Design review of the part built by this model. Coordinates are the model's own, in mm. A direction names the side the tool comes from. Give positions to 0.01 mm unless a question says otherwise; leave off trailing zeros. Write each loop counter-clockwise with the first axis right and the second up, starting at its lowest first coordinate (ties: lowest second). Pieces come first, ordered by that corner, then holes. Notation, with made-up numbers: (62, 20.5) -> (72, 20.5) arc R19 cw to (72, 39.5) -> close; hole circle Ø9 at (43.25, -17). An arc over 180 degrees is marked (long way). Put each result on its own line as item: value. Start each with the question number.
from build123d import *

# Parameters (mm, degrees)
F1_DEPTH        = 12.7
F3_DEPTH        = 25.4
F4_W            = 242.7691146731
F4_H            = 30.0364848226
F5_DEPTH        = 12.7
F6_R            = 14.6387815084
F7_DEPTH        = 25.4
F8_R            = 8.3487757397
F9_DEPTH        = 25.4
F11_DEPTH       = 5.08
F13_DEPTH       = 5.08
F15_D           = 8.8
F15_CSINK_D     = 17.92
F15_CSINK_ANGLE = 90


with BuildPart() as f1:
    # F0 (on Top) → F1 (new body)
    with BuildSketch(Plane.XY):
        with BuildLine():
            Line((-109.5926865071, 0), (109.5926865071, 0))
            ThreePointArc((109.5926865071, 0), (0, 109.5926865071), (-109.5926865071, 0))
        make_face()
    extrude(amount=F1_DEPTH)

    # F2 (on Top) → F3 (join)
    with BuildSketch(Plane.XY):
        with BuildLine():
            Line((-99.2360358279, 0), (99.2360358279, 0))
            ThreePointArc((99.2360358279, 0), (0, 99.2360358279), (-99.2360358279, 0))
        make_face()
    extrude(amount=F3_DEPTH)

    # F4 (on Top) → F5 (cut)
    with BuildSketch(Plane.XY):
        with Locations((-4.4899918139, -4.9826959148)):
            Rectangle(F4_W, F4_H)
    extrude(amount=F5_DEPTH, mode=Mode.SUBTRACT)

    # F6 (on Top) → F7 (join)
    with BuildSketch(Plane.XY):
        Circle(F6_R)
    extrude(amount=F7_DEPTH)

    # F8 (on Top) → F9 (cut)
    with BuildSketch(Plane.XY):
        Circle(F8_R)
    extrude(amount=F9_DEPTH, mode=Mode.SUBTRACT)

    # F10 (on Top) → F11 (cut)
    with BuildSketch(Plane.XY):
        with BuildLine():
            ThreePointArc((81.0422290099, 30.3221999213), (83.5344690722, 31.6522479843), (83.8168430896, 34.4630402733))
            ThreePointArc((83.8168430896, 34.4630402733), (71.7577369395, 55.3515268057), (54.6157974615, 72.3192851046))
            ThreePointArc((54.6157974615, 72.3192851046), (52.4026696923, 72.89779249), (50.4251048932, 71.7480782719))
            Line((50.4251048932, 71.7480782719), (22.4235640904, 35.1450000601))
            ThreePointArc((22.4235640904, 35.1450000601), (22.1166466893, 31.9933659242), (24.806293545, 30.3221999213))
            Line((24.806293545, 30.3221999213), (81.0422290099, 30.3221999213))
        make_face()
        with BuildLine():
            ThreePointArc((-4.9650533663, 33.315884659), (-2.6194064658, 32.1600273833), (-0.2580637548, 33.2834712068))
            Line((-0.2580637548, 33.2834712068), (36.3094015687, 78.8968902074))
            ThreePointArc((36.3094015687, 78.8968902074), (36.8765863049, 81.5111398441), (35.1316920138, 83.538784685))
            ThreePointArc((35.1316920138, 83.538784685), (-1.7558791181, 90.6083948589), (-38.3418575582, 82.1149577688))
            ThreePointArc((-38.3418575582, 82.1149577688), (-39.9894725562, 80.0980697861), (-39.4389206806, 77.5526101127))
            Line((-39.4389206806, 77.5526101127), (-4.9650533663, 33.315884659))
        make_face()
        with BuildLine():
            ThreePointArc((-28.6519128364, 30.3221999213), (-25.9512730857, 32.0158519826), (-26.2999293888, 35.1845032967))
            Line((-26.2999293888, 35.1845032967), (-53.425476113, 69.442529))
            ThreePointArc((-53.425476113, 69.442529), (-55.4614488813, 70.5635354057), (-57.6870926805, 69.8939458642))
            ThreePointArc((-57.6870926805, 69.8939458642), (-70.419089982, 57.0448603864), (-80.3456057092, 41.9231197982))
            ThreePointArc((-80.3456057092, 41.9231197982), (-80.3231983412, 39.1054090847), (-77.9741099322, 37.5492023498))
            ThreePointArc((-77.9741099322, 37.5492023498), (-71.346139634, 35.2966967191), (-66.4208829403, 30.3221999213))
            Line((-66.4208829403, 30.3221999213), (-28.6519128364, 30.3221999213))
        make_face()
    extrude(amount=F11_DEPTH, mode=Mode.SUBTRACT)

    # F12 (on Top) → F13 (cut)
    with BuildSketch(Plane.XY):
        with BuildLine():
            ThreePointArc((-89.5017917801, 37.8877817543), (-64.6761122502, 72.5469175245), (-27.4057276817, 93.2468810649))
            ThreePointArc((-27.4057276817, 93.2468810649), (-25.7155974631, 98.6594259136), (-30.9120716898, 100.9285309146))
            ThreePointArc((-30.9120716898, 100.9285309146), (-70.8203505983, 78.2726163475), (-97.3429498314, 40.8224772259))
            ThreePointArc((-97.3429498314, 40.8224772259), (-94.7015703839, 35.937260015), (-89.5017917801, 37.8877817543))
        make_face()
    extrude(amount=F13_DEPTH, mode=Mode.SUBTRACT)

    # F15 (through all)
    with Locations(Plane(origin=(0, 0, 0), x_dir=(1, 0, 0), z_dir=(0, 0, -1))):
        with Locations((84.3808501959, -22.1120715141), (-79.4403954111, -22.3570616146)):
            CounterSinkHole(F15_D / 2, F15_CSINK_D / 2, counter_sink_angle=F15_CSINK_ANGLE)


solid = f1.part
Q1. Take a section at A-A on y = 4. Give the boundary of the cut face in (x, z).
Q2. To check wall thickness, follow probe 1 along X at (y, z) = (21, 9.75); probe 2 along Y at (x, z) = (0, 11.75); probe 3 along X at (y, z) = (23.5, 23.5). State the ranges of each line that lie inside material, in increasing order. Write a range as from..to.
Q3. Take a section at D-D on y = 52.5. Give the boundary of the cut face in (x, z), then the cut area to 3 significant figures.
Q4. For pin 1 (4 mm diameter, centred on x = -71.5, z = 19, fed in from -Y); pin 2 (10 mm diameter, centred on x = -20.5, z = 4.5, fed in from -Y); pin 3 (12 mm diameter, centred on x = 70.5, z = 20, fed in from +Y); pin 4 (5 mm diameter, centred on y = 11, z = 15, fed in from -X), all flat-tipped, find the tip position at first contact; note any pin that passes through.
Q5. Machinability: for faces 1 (the face through (-1.81, -8.15, 12.52)), 2 (the face through (36.62, 53.7, 2.5)), which of the approach directions +Z, -Z, +X, -X, +Y, -Y give a long, thin tool a straight path to every point of the face, cutting with its end or side? Answer none if there is none.
Q6. Take a section at B-B on z = 14.75. Give the boundary of the cut face in (x, y).
Q7. Mouldability with a two-part tool opening along X and no side actions: class faces 3 (the face through (56, 0, 19)), 4 (the face through (-94.781, 35.968, 2.504)), 5 (the face through (2.182, 99.212, 18.961)) as +X half, -X half, draft (parallel to the pull), parting line (faces both ways), or undercut.
Q8. Take a section at C-C on x = 58. Give the boundary of the cut face in (y, z).
Result:
1. outline: (-99.16, 12.7) -> (-14.08, 12.7) -> (-14.08, 0) -> (-7.33, 0) -> (-7.33, 25.4) -> (-99.16, 25.4) -> close; (7.33, 0) -> (14.08, 0) -> (14.08, 12.7) -> (99.16, 12.7) -> (99.16, 25.4) -> (7.33, 25.4) -> close
2. probe 1: x = -107.56..-83.63, -75.25..80.12, 88.64..107.56
2. probe 2: y = -14.64..-8.35, 8.35..109.59
2. probe 3: x = -96.41..-83.69, -75.19..80.21, 88.56..96.41
3. outline: (-96.2, 0) -> (-91.57, 0) -> (-91.57, 5.08) -> (-81.79, 5.08) -> (-81.79, 0) -> (-73.87, 0) -> (-73.87, 5.08) -> (-40.01, 5.08) -> (-40.01, 0) -> (-19.92, 0) -> (-19.92, 5.08) -> (15.15, 5.08) -> (15.15, 0) -> (35.7, 0) -> (35.7, 5.08) -> (73.87, 5.08) -> (73.87, 0) -> (96.2, 0) -> (96.2, 12.7) -> (84.21, 12.7) -> (84.21, 25.4) -> (-84.21, 25.4) -> (-84.21, 12.7) -> (-96.2, 12.7) -> close
3. area: 3,990 mm^2
4. pin 1: stops at y = 0
4. pin 2: stops at y = 10.04
4. pin 3: stops at y = 75.42
4. pin 4: stops at x = -109.13
5. face 1: +Z, -Z
5. face 2: -Z
6. outline: (-99.24, 0) -> (-14.64, 0) arc R14.64 ccw to (14.64, 0) -> (99.24, 0) arc R99.24 ccw to start; hole circle Ø8.8 at (-79.44, 22.36); hole circle Ø16.7 at (0, 0); hole circle Ø8.8 at (84.38, 22.11)
7. face 3: draft
7. face 4: undercut
7. face 5: parting line
8. outline: (0, 12.7) -> (10.04, 12.7) -> (10.04, 0) -> (30.32, 0) -> (30.32, 5.08) -> (69.63, 5.08) -> (69.63, 0) -> (92.99, 0) -> (92.99, 12.7) -> (80.52, 12.7) -> (80.52, 25.4) -> (0, 25.4) -> close
